from build123d import *

# Parameters (mm, degrees)
F1_DEPTH = 86.36


# Not quite as in the source:
# - a feature of the source that left no trace in its solid (it failed there, or was rolled back) is left out


with BuildPart() as f1:
    # F0 (on Front) → F1 (new body)
    with BuildSketch(Plane.XZ):
        with BuildLine():
            Line((699.6463771647, 476.5957295895), (-1027.3060432158, 476.5957295895))
            ThreePointArc((-1027.3060432158, 476.5957295895), (-1032.2305974455, 474.2546278967), (-1033.5240076617, 468.9575455385))
            Line((-1033.5240076617, 468.9575455385), (-841.4893746376, -457.9787254334))
            Line((-841.4893746376, -457.9787254333), (513.829767704, -457.9787254333))
            Line((513.829767704, -457.9787254333), (705.8643416894, 468.9575459187))
            ThreePointArc((705.8643416894, 468.9575459187), (704.5709312719, 474.2546280473), (699.6463771647, 476.5957295895))
        make_face()
    extrude(amount=F1_DEPTH)


solid = f1.part
Model file for the job. Use its own axes, mm. Give positions to 0.01 mm unless a question says otherwise; leave off trailing zeros. Write each loop counter-clockwise with the first axis right and the second up, starting at its lowest first coordinate (ties: lowest second). Pieces come first, ordered by that corner, then holes. Notation, with made-up numbers: M -10.5,14.5 L 2.5,14.5 A25 cw 2.5,29.5 Z; hole C 66.25,7 d7. An arc over 180 degrees is marked long. One line per item, written item: value. Start each with the question number.
Q1. Saw through at B-B, the plane z = -73. Write the cut outline in (x, y).
Q2. Saw through at A-A, the plane y = -52. Write the cut outline in (x, z).
Q3. Drop flat-ended pins along their axis: pin 1 Ø2 at (y, z) = (-36.5, 168.5) entering from -X (3 decimals); pin 2 Ø4 at (y, z) = (-9.5, 3) entering from +X; pin 3 Ø5 at (y, z) = (-19.5, -285) entering from -X. Give the stop position or say it passes through.
Q4. Probe probe 1 along X at (y, z) = (-23.5, -190); probe 2 along X at (y, z) = (-66, -32.5). List the from-to ranges inside material, lowest first. Write a range as [from, to].
Q5. Saw through at C-C, the plane x = 556.5. Write the cut outline in (y, z), plus the area to 3 significant figures.
Output values:
1. outline: M -921.25,-86.36 L 593.59,-86.36 L 593.59,0 L -921.25,0 Z
2. outline: M -1033.52,468.96 L -841.49,-457.98 L 513.83,-457.98 L 705.86,468.96 A6.35 ccw 699.65,476.6 L -1027.31,476.6 A6.35 ccw Z
3. pin 1: stops at x = -971.485
3. pin 2: stops at x = 609.75
3. pin 3: stops at x = -877.84
4. probe 1: x = [-897.01, 569.35]
4. probe 2: x = [-929.64, 601.98]
5. outline: M -86.36,-252.01 L 0,-252.01 L 0,476.6 L -86.36,476.6 Z
5. area: 62,900 mm²
